Verification items for this drawing (mm, ordinates from the low corner). Round coordinates to 2 decimals unless told otherwise and drop trailing zeros. Loops run counter-clockwise (first coordinate to the right, second up) from the corner with the lowest first, then second, coordinate; pieces in that order, holes last. Notation, with made-up numbers: M 53,82.5 L 59,82.5 A11 ccw 59,97.5 Z; hole C 85.5,3 d6. An arc over 180 degrees is marked long. Answer in a Markdown table with one row per item. Add a question column.
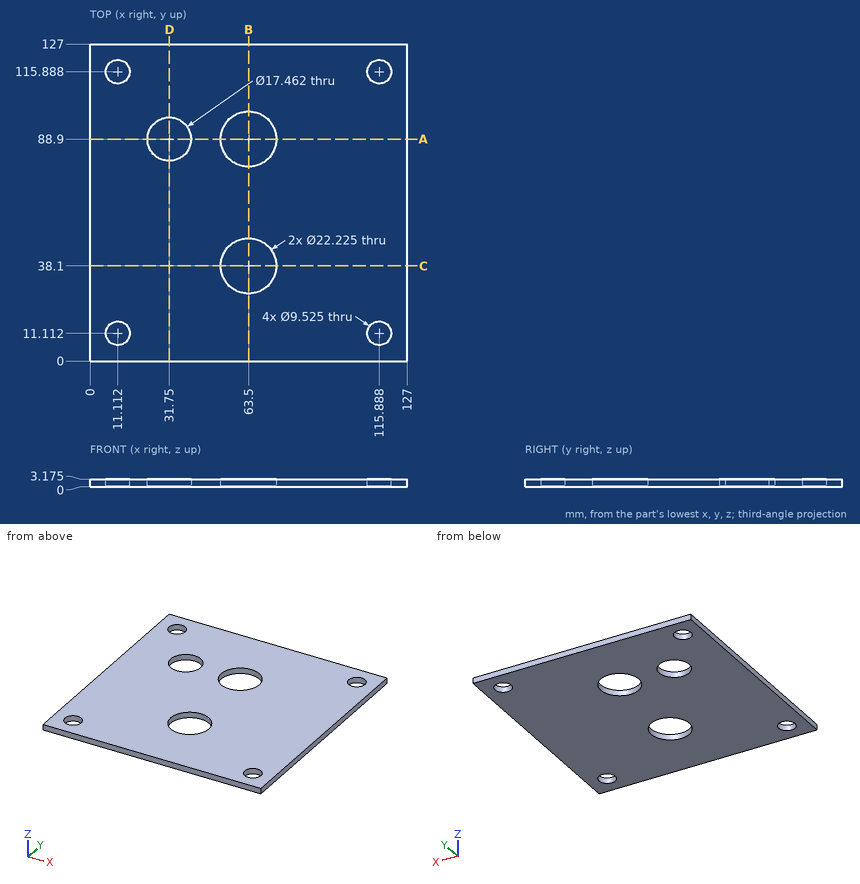
1) Cross-section at C-C, the plane y = 38.1. Record the boundary of the cut face in (x, z) (1 decimal).
2) Cross-section at A-A, the plane y = 88.9. Record the boundary of the cut face in (x, z) (1 decimal), plus the area to 3 significant figures.
3) Cross-section at D-D, the plane x = 31.75. Record the boundary of the cut face in (y, z) (1 decimal), plus the area to 3 significant figures.
4) Thickness scan on L1, parallel to X at y = 116, z = 2.2; L2, parallel to Y at x = 63.5, z = 1.6; L3, parallel to Y at x = 114.5, z = 0.45 (1 decimal). Record the ranges inside material, lowest first. Write a range as [from, to].
5) Go/stop test with a flat-tipped pin: pin 1 (12.5 mm diameter, centred on x = 11.11, y = 11.11, fed in from -Z). Record where the tip stops, or that it passes through.
6) Cross-section at B-B, the plane x = 63.5. Record the boundary of the cut face in (y, z) (1 decimal), plus the area to 3 significant figures.
Worked answers:
| question | item | result |
|---|---|---|
| 1 | outline | M 0,0 L 52.4,0 L 52.4,3.2 L 0,3.2 Z; M 74.6,0 L 127,0 L 127,3.2 L 74.6,3.2 Z |
| 2 | outline | M 0,0 L 23,0 L 23,3.2 L 0,3.2 Z; M 40.5,0 L 52.4,0 L 52.4,3.2 L 40.5,3.2 Z; M 74.6,0 L 127,0 L 127,3.2 L 74.6,3.2 Z |
| 2 | area | 277 mm2 |
| 3 | outline | M 0,0 L 80.2,0 L 80.2,3.2 L 0,3.2 Z; M 97.6,0 L 127,0 L 127,3.2 L 97.6,3.2 Z |
| 3 | area | 348 mm2 |
| 4 | L1 | x = [0, 6.35], [15.87, 111.13], [120.65, 127] |
| 4 | L2 | y = [0, 26.99], [49.21, 77.79], [100.01, 127] |
| 4 | L3 | y = [0, 6.6], [15.7, 111.3], [120.4, 127] |
| 5 | pin 1 | stops at z = 0 |
| 6 | outline | M 0,0 L 27,0 L 27,3.2 L 0,3.2 Z; M 49.2,0 L 77.8,0 L 77.8,3.2 L 49.2,3.2 Z; M 100,0 L 127,0 L 127,3.2 L 100,3.2 Z |
| 6 | area | 262 mm2 |
